Can you work these out from the model? Positions are in its coordinate system, mm. A direction names the side the tool comes from. Round coordinates to 2 decimals unless told otherwise and drop trailing zeros. Order: outer loops, then holes, each group sorted by start corner. A loop starts at its lowest first (then second) coordinate and runs counter-clockwise, first axis right, second up.
Q1. If we section it at B-B (x = -0.75): Please give me the cut outline in (y, z).
Q2. If I drill on line 1 (X direction, y = 0.5, z = -1.75); line 2 (Z direction, x = -2, y = -2.75); line 3 (Z direction, x = 3.25, y = 2.25), over which ranges is the centre line in solid material (lowest first)?
Q3. If we section it at A-A (x = 1.75): Please give me the cut outline in (y, z).
Q4. For faces 1 (the face through (-0.076, 0.009, -3.632)), 2 (the face through (4, 0, -2)), which set-ups out of +Z, -Z, +X, -X, +Y, -Y let a thin tool reach every point of the face, with its end or its side?
Q5. Will these pins go through, and if not, where does the flat tip stop? P1, Ø4, axis at x = -5.5, y = 2.5, coming from the +Z side; P2, Ø2, axis at y = 2.5, z = 3, coming from the -X side.
Autodesk Inventor part; units mm, degrees
ref_plane "YZ Plane" through (0, 0, 0) normal (1, 0, 0) x (0, 1, 0)
ref_plane "XZ Plane" through (0, 0, 0) normal (0, 1, 0) x (-1, 0, 0)
ref_plane "XY Plane" through (0, 0, 0) normal (0, 0, 1) x (1, 0, 0)
sketch "Esquisse1" plane through (0, 0, 0) normal (0, 0, 1) x (1, 0, 0)
  line L0 (-8.8, 0) -> (-8.8, 2.4)
  line L1 (-8.8, 2.4) -> (-7.335, 3.2016)
  line L2 (-8.8, 0) -> (4.7, 0)
  line L3 (4.7, 0) -> (4.7, 1.5)
  line L4 (4.7, 1.5) -> (4, 1.5)
  line L5 (4, 1.5) -> (4, 3)
  line L6 (4, 3) -> (0, 3)
  arc A0 (-4.7886, 2.8) -> (-7.335, 3.2016) centre (-6.535, 0) ccw
  line L7 (-11.5, 0) -> (7.4, 0)
  line L8 (0, -1.7331) -> (0, 10.3984)
  arc A1 (-4.7886, 2.8) -> (-3, 3.5) centre (-6.0528, 8.6653) ccw
  line L9 (-3, 3.5) -> (0, 3.5)
  line L10 (0, 3.5) -> (0, 3)
  dimension "d0" = 13.5
  dimension "d1" = 5.6
  dimension "d2" = 0.7
  dimension "d3" = 3
  dimension "d4" = 6
  dimension "d5" = 6.6
  dimension "d6" = 4.8
  dimension "d7" = 6
  dimension "d11" = 7
  dimension "d14" = 3
  dimension "d15" = 4
  dimension "d61" = 7.335
  dimension "d62" = 6.5351
revolve "Corps" add sketch "Esquisse1" angle 360 about axis through (-8.8, 0, 0) along (1, 0, 0)
fillet "Congé1" radius 0.2 1 edges at (-8.8, -2.4, 0)
thread "Filetage1"
sketch "Esquisse2" plane through (0, 0, 0) normal (1, 0, 0) x (0, 0, -1)
  circle A0 centre (0, 0) radius 3.5
  line L0 (2.0207, 3.5) -> (4.0415, 0)
  line L1 (4.0415, 0) -> (2.0207, -3.5)
  line L2 (2.0207, -3.5) -> (-2.0207, -3.5)
  line L3 (-2.0207, -3.5) -> (-4.0415, 0)
  line L4 (-4.0415, 0) -> (-2.0207, 3.5)
  line L5 (-2.0207, 3.5) -> (2.0207, 3.5)
extrude "Tête" add sketch "Esquisse2" against normal blind 3 contours A0 L0 L1 | A0 L5 L0 | L1 L2 A0 | A0 L4 L5 | L2 L3 A0 | A0 L3 L4
sketch "Esquisse3" plane through (0, 0, 0) normal (0, 1, 0) x (-1, 0, 0)
  line L0 (2.6874, 4.0415) -> (3, 4.0415)
  line L1 (3, 4.0415) -> (3, 3.5)
  line L2 (3, 3.5) -> (2.6874, 4.0415)
  line L3 (0.3126, 4.0415) -> (0, 4.0415)
  line L4 (0, 4.0415) -> (0, 3.5)
  line L5 (0, 3.5) -> (0.3126, 4.0415)
  line L6 (3.6, 0) -> (-0.6, 0)
  line L7 (0, 4.0415) -> (0, 2.0207)
  line L8 (0, 4.0415) -> (3, 4.0415)
  line L9 (3, 3.0311) -> (3, 4.0415)
  dimension "d19" = 3.5
  dimension "d20" = 3.5
  dimension "d21" = 30
  dimension "d22" = 30
revolve "Chanfrein1" cut sketch "Esquisse3" angle 360 about axis through (-10, 0, 0) along (1, 0, 0)
chamfer "Chanfrein2" distance 0.6135 angle 45 1 edges at (4, -3, 0) measured on face at (4, 2.4564, -0.359)
equation "\"d17\" = KOH"
equation "\"d8\" = RR"
equation "\"d9\" = NLG - GAL"
equation "\"d23\" = -0.5 * GD1 + 0.5 * NND"
equation "\"d59\" = -0.5 * GD1 + 0.5 * NND"
equation "\"d0\" = GL"
equation "\"d1\" = KGB2"
equation "\"d2\" = PHH"
equation "\"d3\" = 0.5 * NND"
equation "\"d4\" = NND"
equation "\"d5\" = KR"
equation "\"d6\" = KGB1"
equation "\"d7\" = RBN"
equation "\"d11\" = SW"
equation "\"d14\" = KOH"
equation "\"d15\" = NLG"
equation "\"d19\" = 0.5 * SW"
equation "\"d20\" = 0.5 * SW"
equation "\"NLG\" = 4"
equation "\"GL\" = 13.5"
equation "\"NND\" = 6"
equation "\"KGB1\" = 4.8"
equation "\"KGB2\" = 5.6"
equation "\"VERS\" = 0.8"
equation "\"KR\" = 6.6"
equation "\"RBN\" = 6"
equation "\"SW\" = 7"
equation "\"KOH\" = 3"
equation "\"GAL\" = 0.61345 * PTC"
equation "\"FAWI\" = 45deg"
equation "\"PHH\" = 0.7"
equation "\"GD1\" = THREADDIA - 1.2269 * PTC"
equation "\"RR\" = 0.2"
equation "\"GUL\" = 0.61345 * PTC"
equation "\"DULO\" = 1.5"
equation "\"PTC\" = 1"
equation "\"GEL\" = 4"
equation "\"THREADDIA\" = 6"
equation "\"TOA\" = 30deg"
properties part number "JIS B 1575 - M 6 F" material "Acier doux"
Solution:
1. outline: (-3.5, -2.02) - (0, -4.04) - (3.5, -2.02) - (3.5, 2.02) - (0, 4.04) - (-3.5, 2.02) - close
2. line 1: x = -8.8 to 4
2. line 2: z = -2.45 to 2.45
2. line 3: z = -1.98 to 1.98
3. outline: circle Ø6 at (0, 0)
4. face 1: -Z, +X
4. face 2: +X
5. P1: stops at z = 3.22
5. P2: stops at x = -7.88
